Input: dimensioned drawing with shaded views. Units: mm. Origin: part minimum x, y, z. Round coordinates to 2 decimals unless told otherwise and drop trailing zeros. Loops run counter-clockwise (first coordinate to the right, second up) from the corner with the lowest first, then second, coordinate; pieces in that order, holes last.
Item 1: First-contact query: P1, Ø0.6, axis at x = 65, y = 0.5, coming from the -Z side; P2, Ø0.6, axis at x = 74.5, y = 1, coming from the +Z side; P3, Ø4, axis at x = 17, z = 12, coming from the -Y side. Flat tips, straight axial feed; report the tip coordinate or a pass-through.
Item 2: Section query B-B on z = 29. Return loops of the section in (x, y).
Item 3: Section query C-C on y = 1.15. Return loops of the section in (x, z).
Item 4: Section query D-D on z = 8. Return loops of the section in (x, y).
Item 5: Pull-direction query (Z, two-part tool) for the marked faces 1 and 2; classes: released by +Z, released by -Z, zero draft, split by the parting line, or undercut.
Item 6: Ray query, L1, parallel to Z at x = 46, y = 2.65; L2, parallel to Z at x = 90, y = 0.3; L3, parallel to X at y = 2.2, z = 43.5. Return the intervals inside material, ascending.
Item 7: Section query A-A on x = 85. Return loops of the section in (y, z), then the cut area to 3 significant figures.
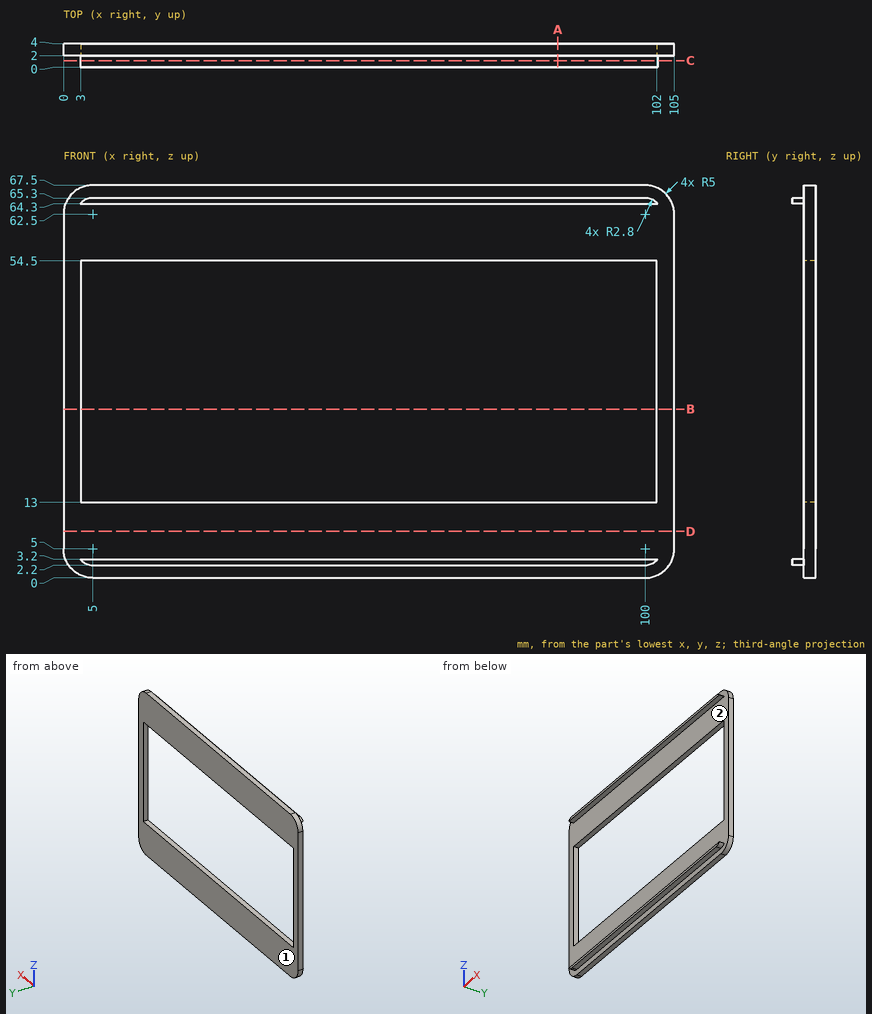
Data:
1. P1: stops at z = 2.2
1. P2: stops at z = 65.3
1. P3: stops at y = 2
2. outline: (0, 2) - (3, 2) - (3, 4) - (0, 4) - close; (102, 2) - (105, 2) - (105, 4) - (102, 4) - close
3. outline: (2.86, 3.2) arc R2.8 ccw to (5, 2.2) - (100, 2.2) arc R2.8 ccw to (102.14, 3.2) - close; (2.86, 64.3) - (102.14, 64.3) arc R2.8 ccw to (100, 65.3) - (5, 65.3) arc R2.8 ccw to start
4. outline: (0, 2) - (105, 2) - (105, 4) - (0, 4) - close
5. face 1: zero draft
5. face 2: undercut
6. L1: z = 0 to 13, 54.5 to 67.5
6. L2: z = 2.2 to 3.2, 64.3 to 65.3
6. L3: x = 0 to 3, 102 to 105
7. outline: (0, 2.2) - (2, 2.2) - (2, 0) - (4, 0) - (4, 13) - (2, 13) - (2, 3.2) - (0, 3.2) - close; (0, 64.3) - (2, 64.3) - (2, 54.5) - (4, 54.5) - (4, 67.5) - (2, 67.5) - (2, 65.3) - (0, 65.3) - close
7. area: 56.0 mm2
